Geometry: see drawing. Coordinates: mm, zero at the bounding-box minimum. A direction names the side the tool comes from. Coordinates: 2 decimals unless noted, no trailing zeros. Loops run counter-clockwise (first coordinate to the right, second up) from the corner with the lowest first, then second, coordinate; pieces in that order, holes last. Notation, with made-up numbers: M 19.5,38.5 L 27.5,38.5 A14 cw 27.5,43.5 Z; hole C -13,3 d1. An arc over 180 degrees is marked long. One line per question, with ' | ' between items. Start each with the question number.
1. Section query A-A, the plane x = 19.75. Output: boundary loops of the cut face in (y, z), and give its area (3 significant figures).
2. Pin query (flat end, axial travel): P1, Ø4, axis at y = 11.5, z = 12, coming from the +X side; P2, Ø2, axis at y = 12.5, z = 13, coming from the -X side; P3, Ø2, axis at x = 12, y = 20.5, coming from the +Z side. Return the tip coordinate at first contact, or that it passes through.
3. Section query B-B, the plane z = 11. Output: boundary loops of the cut face in (x, y), and give its area (3 significant figures).
4. Access query for the marked faces 1, 2, 3 and 4. Directions: +Z, -Z, +X, -X, +Y, -Y. A direction counts if a zero-diameter tool reaches every point of the face in a straight line with its end or side. Return the directions, or none.
5. Section query C-C, the plane y = 10. Output: boundary loops of the cut face in (x, z).
6. Mould query, pull axis X, two halves, no side actions, for the marked faces 5, 6 and 7. Classes: pulls with the +X half, pulls with the -X half, needs draft (parallel to the pull), parting line crosses it, or undercut.
7. Ray query, probe 1 along X at (y, z) = (18, 20); probe 2 along X at (y, z) = (8.25, 18). Return the intervals inside material, ascending.
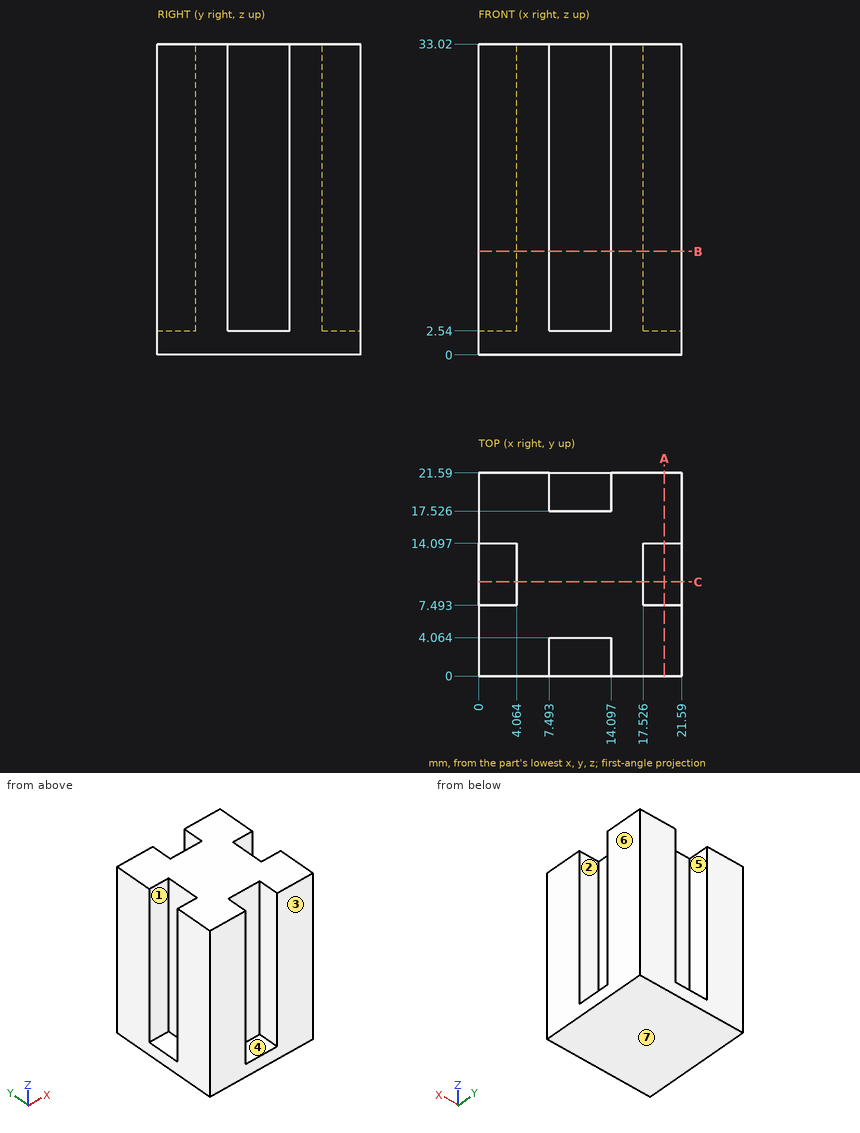
Taken from the geometry:
1) outline: M 0,0 L 21.59,0 L 21.59,33.02 L 14.1,33.02 L 14.1,2.54 L 7.49,2.54 L 7.49,33.02 L 0,33.02 Z | area: 512 mm^2
2) P1: x = 17.53 | P2: x = 4.06 | P3: z = 2.54
3) outline: M 0,0 L 7.49,0 L 7.49,4.06 L 14.1,4.06 L 14.1,0 L 21.59,0 L 21.59,7.49 L 17.53,7.49 L 17.53,14.1 L 21.59,14.1 L 21.59,21.59 L 14.1,21.59 L 14.1,17.53 L 7.49,17.53 L 7.49,21.59 L 0,21.59 L 0,14.1 L 4.06,14.1 L 4.06,7.49 L 0,7.49 Z | area: 359 mm^2
4) face 1: +Z, -X | face 2: +Z, +X | face 3: +Z, -Z, +X, -X, -Y | face 4: +Z, -Y
5) outline: M 0,0 L 21.59,0 L 21.59,2.54 L 17.53,2.54 L 17.53,33.02 L 4.06,33.02 L 4.06,2.54 L 0,2.54 Z
6) face 5: undercut | face 6: pulls with the +X half | face 7: needs draft
7) probe 1: 0 to 7.49, 14.1 to 21.59 | probe 2: 4.06 to 17.53
